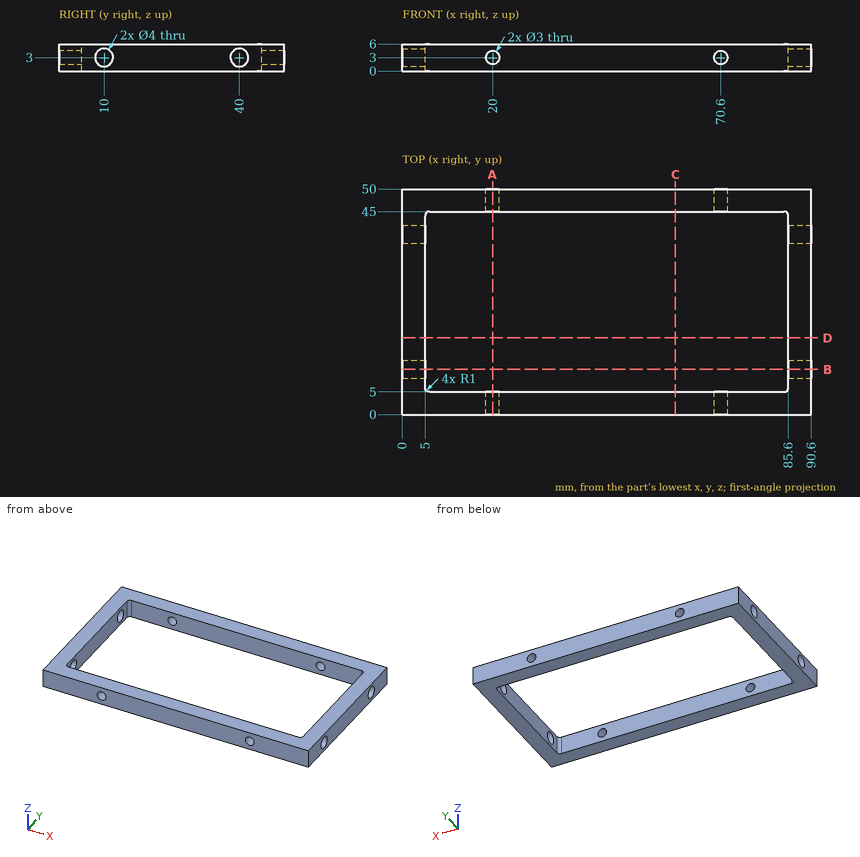
Design review of the part shown in the three views and the two pictorial views. Dimensions are in mm from the part's minimum x, y and z. Round coordinates to 2 decimals unless told otherwise and drop trailing zeros. Loops run counter-clockwise (first coordinate to the right, second up) from the corner with the lowest first, then second, coordinate; pieces in that order, holes last. Notation, with made-up numbers: M 72.25,84 L 117.25,84 A6 ccw 117.25,95 Z; hole C 50.25,88.5 d9. An arc over 180 degrees is marked long. Put each result on its own line as item: value.
Q1. For pin 1 (1 mm diameter, centred on y = 25.5, z = 2, fed in from -X); pin 2 (2.5 mm diameter, centred on y = 10, z = 3, fed in from -X), all flat-tipped, find the tip position at first contact; note any pin that passes through.
Result set:
pin 1: stops at x = 0
pin 2: passes through
Q2. Consider section B-B, the plane y = 10. Give the boundary of the cut face in (x, z).
Result set:
outline: M 0,0 L 5,0 L 5,1 L 0,1 Z; M 0,5 L 5,5 L 5,6 L 0,6 Z; M 85.6,0 L 90.6,0 L 90.6,1 L 85.6,1 Z; M 85.6,5 L 90.6,5 L 90.6,6 L 85.6,6 Z
Q3. To check wall thickness, follow L1, parallel to X at y = 46.15, z = 3; L2, parallel to Y at x = 87.4, z = 3; L3, parallel to X at y = 44, z = 3.85. State the ranges of each line that lie inside material, in increasing order.
Result set:
L1: x = 0 to 18.5, 21.5 to 69.1, 72.1 to 90.6
L2: y = 0 to 8, 12 to 38, 42 to 50
L3: x = 0 to 5, 85.6 to 90.6
Q4. Consider section D-D, the plane y = 17. Give the boundary of the cut face in (x, z), then the cut area to 3 significant figures.
Result set:
outline: M 0,0 L 5,0 L 5,6 L 0,6 Z; M 85.6,0 L 90.6,0 L 90.6,6 L 85.6,6 Z
area: 60.0 mm²
Q5. Consider section C-C, the plane x = 60.5. Give the boundary of the cut face in (y, z), then the cut area to 3 significant figures.
Result set:
outline: M 0,0 L 5,0 L 5,6 L 0,6 Z; M 45,0 L 50,0 L 50,6 L 45,6 Z
area: 60.0 mm²
Q6. Consider section A-A, the plane x = 20. Give the boundary of the cut face in (y, z).
Result set:
outline: M 0,0 L 5,0 L 5,1.5 L 0,1.5 Z; M 0,4.5 L 5,4.5 L 5,6 L 0,6 Z; M 45,0 L 50,0 L 50,1.5 L 45,1.5 Z; M 45,4.5 L 50,4.5 L 50,6 L 45,6 Z
